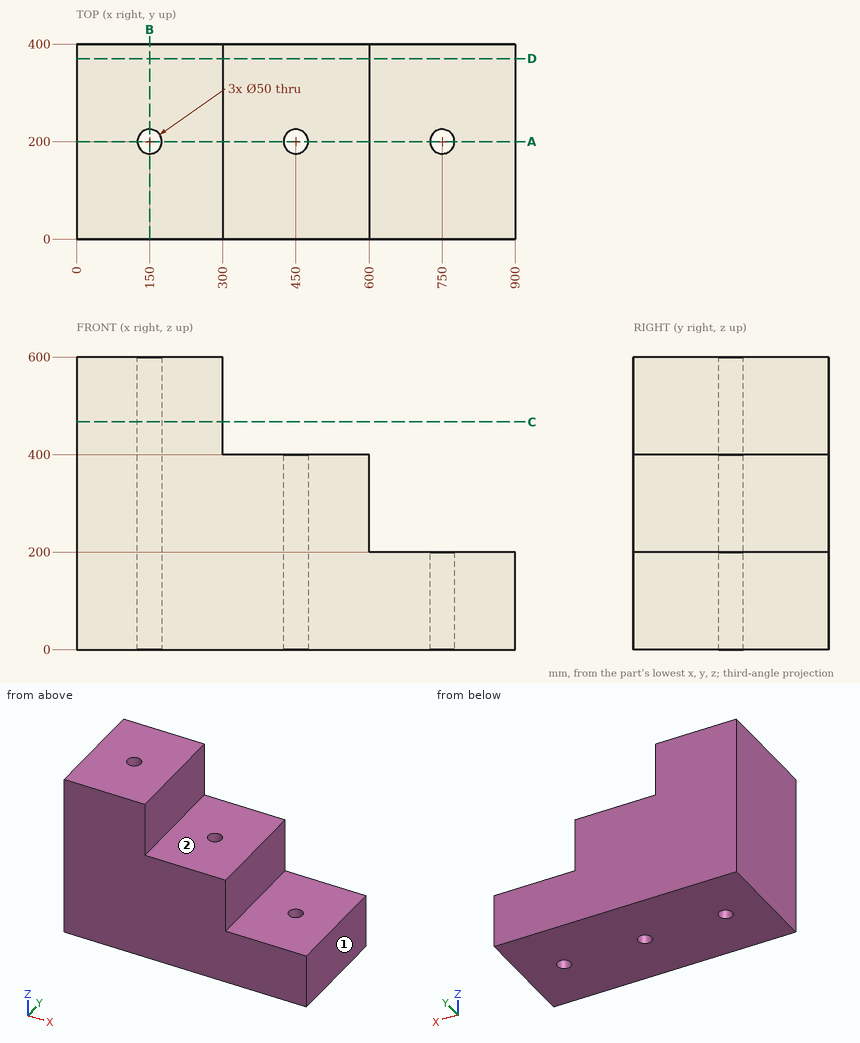
Print and shaded views of the part. All mm, measured from the part's lowest x, y and z. A direction names the side the tool comes from. Coordinates: 2 decimals unless noted, no trailing zeros. Loops run counter-clockwise (first coordinate to the right, second up) from the corner with the lowest first, then second, coordinate; pieces in that order, holes last. Notation, with made-up numbers: (82.25, 56.5) - (117.25, 56.5) arc R28 cw to (117.25, 78.5) - close; hole circle Ø3 at (20.5, 53.5). An arc over 180 degrees is marked (long way). Use one line per item in the form item = value. Start each with the question number.
1) Drill centre lines: L1, parallel to X at y = 202.5, z = 99; L2, parallel to X at y = 202, z = 461; L3, parallel to Y at x = 150, z = 333. Where is each one in solid material? Low to high. Write a range as from..to.
2) Band-saw the part on C-C (z = 467). Give the cut face in (x, y), and give its area (3 significant figures).
3) Band-saw the part on A-A (y = 200). Give the cut face in (x, z), and give its area (3 significant figures).
4) Band-saw the part on D-D (y = 370). Give the cut face in (x, z), and give its area (3 significant figures).
5) Tool access for the marked faces 1 and 2: list every direction of +Z, -Z, +X, -X, +Y, -Y with a clear straight run to the whole face (end or side of a thin tool).
6) Flat gauge pins, fed straight in: pin 1 (5 mm diameter, centred on x = 161, z = 332, fed in from -Y); pin 2 (8 mm diameter, centred on y = 40.5, z = 455.5, fed in from +X); pin 3 (6 mm diameter, centred on x = 444.5, y = 354, fed in from +Z). Where does each tip first touch, or does it go through?
7) Band-saw the part on B-B (x = 150). Give the cut face in (y, z).
Check values:
q1.L1 = 0..125.13, 174.87..425.13, 474.87..725.13, 774.87..900
q1.L2 = 0..125.08, 174.92..300
q1.L3 = 0..175, 225..400
q2.outline = (0, 0) - (300, 0) - (300, 400) - (0, 400) - close; hole circle Ø50 at (150, 200)
q2.area = 118,000 mm2
q3.outline = (0, 0) - (125, 0) - (125, 600) - (0, 600) - close; (175, 0) - (425, 0) - (425, 400) - (300, 400) - (300, 600) - (175, 600) - close; (475, 0) - (725, 0) - (725, 200) - (600, 200) - (600, 400) - (475, 400) - close; (775, 0) - (900, 0) - (900, 200) - (775, 200) - close
q3.area = 300,000 mm2
q4.outline = (0, 0) - (900, 0) - (900, 200) - (600, 200) - (600, 400) - (300, 400) - (300, 600) - (0, 600) - close
q4.area = 360,000 mm2
q5.face_1 = +Z, -Z, +X, +Y, -Y
q5.face_2 = +Z, +X, +Y, -Y
q6.pin_1 = 0
q6.pin_2 = 300
q6.pin_3 = 400
q7.outline = (0, 0) - (175, 0) - (175, 600) - (0, 600) - close; (225, 0) - (400, 0) - (400, 600) - (225, 600) - close
